from build123d import *

# Parameters (mm, degrees)
EXTRUDE_1_DEPTH     = 3
CUT_EXTRUDE_1_REACH = 94.582
SKETCH_2_R          = 1.7
FILLET_1_R          = 1


with BuildPart() as part:
    # 草图1 → 凸台-拉伸1 (new body)
    with BuildSketch(Plane(origin=(0, 0, 0), x_dir=(1, 0, 0), z_dir=(0, 1, 0))):
        with BuildLine():
            Line((2.5, 0), (2.5, 90))
            ThreePointArc((2.5, 90), (0, 92.5), (-2.5, 90))
            Line((-2.5, 90), (-2.5, 0))
            ThreePointArc((-2.5, 0), (0, -2.5), (2.5, 0))
        make_face()
    extrude(amount=EXTRUDE_1_DEPTH)

    # 草图2 → 切除-拉伸1 (cut, up to next)
    with BuildSketch(Plane(origin=(0, 3, 0), x_dir=(1, 0, 0), z_dir=(0, 1, 0)), mode=Mode.PRIVATE) as cut_extrude_1_sk1:
        with Locations(Location((0, 0, 0), (0, 0, 270))):
            Circle(SKETCH_2_R)
    cut_extrude_1_tool1 = extrude(cut_extrude_1_sk1.sketch, amount=-CUT_EXTRUDE_1_REACH, mode=Mode.PRIVATE) & part.part
    # 草图2 → 切除-拉伸1 (cut, up to next)
    with BuildSketch(Plane(origin=(0, 3, 0), x_dir=(1, 0, 0), z_dir=(0, 1, 0)), mode=Mode.PRIVATE) as cut_extrude_1_sk2:
        with Locations(Location((0, 90, 0), (0, 0, 270))):
            Circle(SKETCH_2_R)
    cut_extrude_1_tool2 = extrude(cut_extrude_1_sk2.sketch, amount=-CUT_EXTRUDE_1_REACH, mode=Mode.PRIVATE) & part.part
    add(cut_extrude_1_tool1.solids().sort_by_distance((0, 3, 0))[0], mode=Mode.SUBTRACT)
    add(cut_extrude_1_tool2.solids().sort_by_distance((0, 3, -90))[0], mode=Mode.SUBTRACT)

    # 圆角1
    fillet_1_edges = [part.edges().sort_by_distance(p)[0] for p in [
        (-2.5, 0, -45),
        (-2.5, 3, -45),
        (2.5, 0, -45),
        (2.5, 3, -45),
    ]]
    fillet(fillet_1_edges, radius=FILLET_1_R)


solid = part.part
Model file for the job. Use its own axes, mm. Coordinates: 2 decimals unless noted, no trailing zeros. Order: outer loops, then holes, each group sorted by start corner. A loop starts at its lowest first (then second) coordinate and runs counter-clockwise, first axis right, second up. Notation, with made-up numbers: (-3.75, 58.5) -> (33.25, 58.5) arc R7 ccw to (33.25, 66.5) -> close; hole circle Ø7 at (-34, 85). An arc over 180 degrees is marked (long way). Return JSON: item names as keys, results as strings. Group by question number.
Item 1: Wall check: line 1 along Z through (x, y) = (0, 0.8); line 2 along X through (y, z) = (2.15, -90); line 3 along Z through (x, y) = (-0.8, 2.7). Give the ranges that are in metal, low to high. Write a range as [from, to].
Item 2: Flat gauge pin, fed straight in: P1, Ø2, axis at x = 0, z = 0, coming from the +Y side. Where does the tip first touch, or does it go through?
Item 3: Pull direction Z, two halves, no side cores. Call faces 1 (the cylindrical face through (-0.1, 1.5, 2.5)), 2 (the cylindrical face through (0.1, 1.5, -92.5)), 3 (the cylindrical face through (0.07, 1.52, -91.7)): pulls with the +Z half, pulls with the -Z half, needs draft (parallel to the pull), parting line crosses it, or undercut.
Item 4: Saw through at A-A on z = -72.5. Write the cut outline in (x, y), then the cut area to 3 significant figures.
Values found:
{
 "1": {"line 1": "z = [-92.48, -91.7], [-88.3, -1.7], [1.7, 2.48]", "line 2": "x = [-2.49, -1.7], [1.7, 2.49]", "line 3": "z = [-92.09, -91.5], [-88.5, -1.5], [1.5, 2.09]"},
 "2": {"P1": "passes through"},
 "3": {"face 1": "pulls with the +Z half", "face 2": "pulls with the -Z half", "face 3": "undercut"},
 "4": {"outline": "(-2.5, 1) arc R1 ccw to (-1.5, 0) -> (1.5, 0) arc R1 ccw to (2.5, 1) -> (2.5, 2) arc R1 ccw to (1.5, 3) -> (-1.5, 3) arc R1 ccw to (-2.5, 2) -> close", "area": "14.1 mm2"}
}
